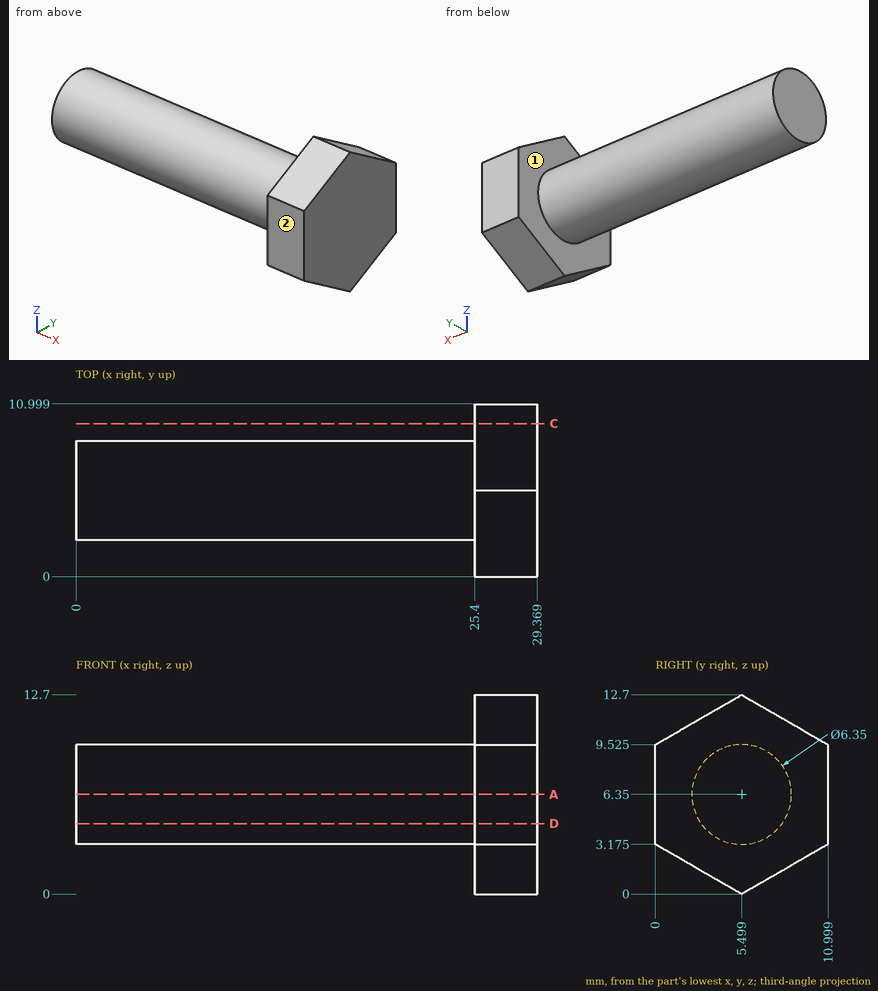
Here's the drawing with two shaded views (mm, measured from the low corner). I have some questions. A direction names the side the tool comes from. Coordinates: 2 decimals unless noted, no trailing zeros. Order: outer loops, then holes, each group sorted by start corner. A loop starts at its lowest first (then second) coordinate and runs counter-clockwise, first axis right, second up.
Item 1: For P1, Ø6, axis at x = 8.5, z = 5.5, coming from the +Y side, with a flat end and sliding along its axis, tell me the tip position at first contact or that it passes through.
Result sheet:
P1: stops at y = 8.67
Item 2: If we section it at A-A on z = 6.35: List the corners of the cut face in (x, y) for me (1 decimal), plus the area to 3 significant figures.
Result sheet:
outline: (0, 2.3) - (25.4, 2.3) - (25.4, 0) - (29.4, 0) - (29.4, 11) - (25.4, 11) - (25.4, 8.7) - (0, 8.7) - close
area: 205 mm2
Item 3: I need wall thicknesses on line 1 (X direction, y = 8.75, z = 7.5); line 2 (Y direction, x = 10, z = 6.5); line 3 (Z direction, x = 19.75, y = 3). Which ranges of each line are inside material? Lowest first, please.
Result sheet:
line 1: x = 25.4 to 29.37
line 2: y = 2.33 to 8.67
line 3: z = 4.39 to 8.31
Item 4: If we section it at D-D on z = 4.5: List the corners of the cut face in (x, y) for me.
Result sheet:
outline: (0, 2.92) - (25.4, 2.92) - (25.4, 0) - (29.37, 0) - (29.37, 11) - (25.4, 11) - (25.4, 8.08) - (0, 8.08) - close
Item 5: If we section it at C-C on y = 9.75: List the corners of the cut face in (x, z) for me.
Result sheet:
outline: (25.4, 2.45) - (29.37, 2.45) - (29.37, 10.25) - (25.4, 10.25) - close
Item 6: For the marked faces 1 and 2, which set-ups out of +Z, -Z, +X, -X, +Y, -Y let a thin tool reach every point of the face, with its end or its side?
Result sheet:
face 1: -X
face 2: +Z, -Z, +X, -X, -Y
